from build123d import *

# Parameters (mm, degrees)
CORTE_EXTRUS_O3_DEPTH      = 92.484637542
CORTE_EXTRUS_O3_DEPTH_BACK = 92.484637542
ESBO_O2_R                  = 2.5


with BuildPart() as part:
    # Esboço1 → Revolução1 (revolve)
    with BuildSketch(Plane.XY, mode=Mode.PRIVATE) as revolu_o1_sk:
        with BuildLine():
            Line((-14.5288, 17.78), (-17.4625, 17.78))
            Line((-17.4625, 17.78), (-17.4625, 13.5001))
            Line((-17.4625, 13.5001), (17.4625, 13.5001))
            Line((17.4625, 13.5001), (17.4625, 17.78))
            Line((17.4625, 17.78), (14.5288, 17.78))
            Line((14.5288, 17.78), (14.5288, 19.05))
            Line((14.5288, 19.05), (8.971561034, 19.53619541))
            ThreePointArc((8.971561034, 19.53619541), (4.843288911, 21.572033925), (3.175, 25.862031743))
            Line((3.175, 25.862031743), (3.175, 50.601191018))
            ThreePointArc((3.175, 50.601191018), (4.843288911, 54.891188837), (8.971561034, 56.927027351))
            Line((8.971561034, 56.927027351), (15.875, 57.531))
            Line((15.875, 57.531), (15.875, 63.5))
            Line((15.875, 63.5), (-15.875, 63.5))
            Line((-15.875, 63.5), (-15.875, 57.531))
            Line((-15.875, 57.531), (-8.971561034, 56.927027351))
            ThreePointArc((-8.971561034, 56.927027351), (-4.843288911, 54.891188837), (-3.175, 50.601191018))
            Line((-3.175, 50.601191018), (-3.175, 25.862031743))
            ThreePointArc((-3.175, 25.862031743), (-4.843288911, 21.572033925), (-8.971561034, 19.53619541))
            Line((-8.971561034, 19.53619541), (-14.5288, 19.05))
            Line((-14.5288, 19.05), (-14.5288, 17.78))
        make_face()
    revolve(revolu_o1_sk.sketch.rotate(Axis((-17.4625, 0, 0), (1, 0, 0)), 270), axis=Axis((-17.4625, 0, 0), (1, 0, 0)))

    # Esboço2 → Corte-extrusão3 (cut, two sides: drawn at the far end of the back side and taken through both)
    with BuildSketch(Plane(origin=(0, 0, 0), x_dir=(0, 0, -1), z_dir=(1, 0, 0)).offset(-CORTE_EXTRUS_O3_DEPTH_BACK)):
        with Locations((0, 38)):
            Circle(ESBO_O2_R)
        with Locations((22.335839587, 30.742645786)):
            Circle(ESBO_O2_R)
        with Locations((36.140147619, 11.742645786)):
            Circle(ESBO_O2_R)
        with Locations((36.140147619, -11.742645786)):
            Circle(ESBO_O2_R)
        with Locations((22.335839587, -30.742645786)):
            Circle(ESBO_O2_R)
        with Locations((0, -38)):
            Circle(ESBO_O2_R)
        with Locations((-22.335839587, -30.742645786)):
            Circle(ESBO_O2_R)
        with Locations((-36.140147619, -11.742645786)):
            Circle(ESBO_O2_R)
        with Locations((-36.140147619, 11.742645786)):
            Circle(ESBO_O2_R)
        with Locations((-22.335839587, 30.742645786)):
            Circle(ESBO_O2_R)
    extrude(amount=CORTE_EXTRUS_O3_DEPTH + CORTE_EXTRUS_O3_DEPTH_BACK, mode=Mode.SUBTRACT)


solid = part.part
Input: part model. Units: mm. Frame: model coordinates. A direction names the side the tool comes from. Round coordinates to 2 decimals unless told otherwise and drop trailing zeros. Answer as a JSON object with one key per item and string values. Group by question number.
(1) Reachability of faces 4 (the face through (-0.04, -40.44, 0.54)), 5 (the face through (-14.529, 9, 16)), 6 (the face through (3.175, 23.2, -12)) from +Z, -Z, +X, -X, +Y, -Y: full face, straight path, thin tool, end or side. Return the list, or none.
(2) Cut plane A-A (x = -1). Count the separate pieces of the cut face and the enclosed holes in it, then the cut area to 3 significant figures.
(3) Material intervals for probe 1 along Z at (x, y) = (-7, 1.5); probe 2 along Y at (x, z) = (8, 7.5); probe 3 along Y at (x, z) = (-8, 0), sorted ascending. Write a range as from..to.
(4) Draft query along Y for faces 1 (the face through (15.875, 57, -10)), 2 (the face through (-0.044, 11.853, -33.643)), 3 (the face through (-0.22, -61.99, 13.77)). Return one class per face: released by +Y, released by -Y, zero draft, split by the parting line, or undercut.
(5) Pin query (flat end, axial travel): P1, Ø12, axis at x = -3.5, z = 39, coming from the +Y side; P2, Ø10, axis at x = -7, y = -42, coming from the +Z side; P3, Ø6.5, axis at y = 30.74, z = -22.34, coming from the +X side (3 decimals). Return the tip coordinate at first contact, or that it passes through.
Here are the results:
{
 "1": {"face 4": "+X, -X", "face 5": "-X", "face 6": "+X"},
 "2": {"separate pieces": "1", "enclosed holes": "11", "area": "11,900 mm^2"},
 "3": {"probe 1": "z = -63.48..-56.41, -19.98..-13.42, 13.42..19.98, 56.41..63.48", "probe 2": "y = -63.06..-56.27, -18.21..-11.23, 11.23..18.21, 56.27..63.06", "probe 3": "y = -63.5..-56.77, -19.7..-13.5, 13.5..19.7, 56.77..63.5"},
 "4": {"face 1": "zero draft", "face 2": "undercut", "face 3": "split by the parting line"},
 "5": {"P1": "stops at y = 54.25", "P2": "stops at z = 51.61", "P3": "stops at x = 3.175"}
}
